CAD build for the part. Positions are in the model's coordinates, mm. Give positions to 0.01 mm unless a question says otherwise; leave off trailing zeros. Write each loop counter-clockwise with the first axis right and the second up, starting at its lowest first coordinate (ties: lowest second). Pieces come first, ordered by that corner, then holes. Notation, with made-up numbers: (64, -7.75) - (121, -7.75) arc R24 cw to (121, 27.25) - close; hole circle Ø10 at (-21.5, 80.5). An arc over 180 degrees is marked (long way). Answer as a JSON object with one key per item and string values.
from build123d import *

# Parameters (mm, degrees)
F0_R     = 1
F1_DEPTH = 111.4
F2_W     = 2
F2_H     = 1
F3_DEPTH = 2.5
F6_R     = 0.4445
F7_DEPTH = 25


# Not quite as in the source:
# - a feature names something its author has since deleted; it is built from what else it names


with BuildPart() as f1:
    # F0 (on Right) → F1 (new body)
    with BuildSketch(Plane.YZ):
        Circle(F0_R)
    extrude(amount=F1_DEPTH)

    # F2 (on Front) → F3 (cut, symmetric)
    with BuildSketch(Plane.XZ):
        with Locations((90.6, -1.3)):
            Rectangle(F2_W, F2_H)
    extrude(amount=F3_DEPTH, both=True, mode=Mode.SUBTRACT)

    # F4 (on Front) → F5 (revolve, cut)
    with BuildSketch(Plane.XZ):
        Polygon((111.4, -0.8), (111.4, 0), (107.8, 0), (108.4, -0.6), (111.2, -0.6), align=None)
        Polygon((0.2, -0.6), (3, -0.6), (3.6, 0), (0, 0), (0, -0.8), align=None)
    revolve(axis=Axis((55.7, 0, 0), (1, 0, 0)), mode=Mode.SUBTRACT)

    # F6 (on face) → F7 (cut)
    with BuildSketch(Plane(origin=(0, 0, -0.8), x_dir=(1, 0, 0), z_dir=(0, 0, -1))):
        with Locations((90.6, 0)):
            Circle(F6_R)
    extrude(amount=-F7_DEPTH, mode=Mode.SUBTRACT)


solid = f1.part
(1) Saw through at A-A, the plane x = 52. Give the cut face in (y, z).
Answer key:
{"outline": "circle Ø2 at (0, 0)"}
(2) Probe L1, parallel to X at y = -0.25, z = -0.9; L2, parallel to Y at x = 90.6, z = -0.05; L3, parallel to Z at x = 64, y = -0.9. List the from-to ranges inside material, lowest first. Write a range as [from, to].
Answer key:
{"L1": "x = [0, 89.6], [91.6, 111.4]", "L2": "y = [-1, -0.44], [0.44, 1]", "L3": "z = [-0.44, 0.44]"}
(3) Flat gauge pins, fed straight in: P1, Ø0.7, axis at y = 0, z = 0, coming from the +X side; P2, Ø1.1, axis at y = 0, z = 0, coming from the +X side. Where does each tip first touch, or does it go through?
Answer key:
{"P1": "stops at x = 108.15", "P2": "stops at x = 108.35"}
